Geometry check sheet. Reference: the model listing, model coordinates, mm. Face numbers are marked on the shaded views. A direction names the side the tool comes from. Give positions to 0.01 mm unless a question says otherwise; leave off trailing zeros. Write each loop counter-clockwise with the first axis right and the second up, starting at its lowest first coordinate (ties: lowest second). Pieces come first, ordered by that corner, then holes. Notation, with made-up numbers: M 5.5,86.25 L 27.5,86.25 A16 ccw 27.5,100.25 Z; hole C 73.5,26.5 d11. An arc over 180 degrees is marked long. Write each question's results on one line, items separated by ' | '.
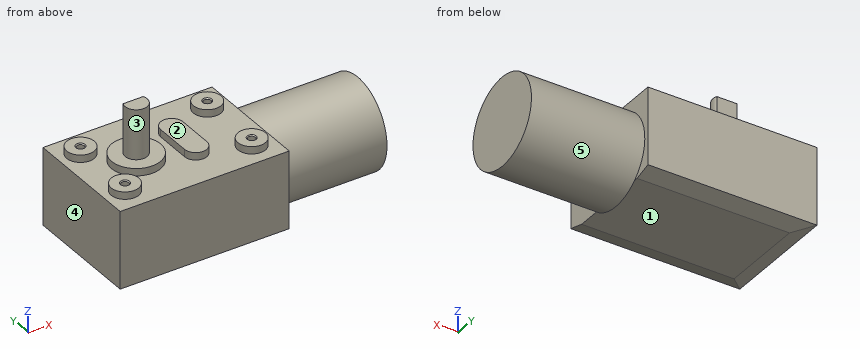
Autodesk Inventor part; units mm, degrees
ref_plane "Arbeitsebene1" through (-28.07, 15.935, 0) normal (-1, 0, 0) x (0, 0, 1)
ref_plane "YZ Plane" through (0, 0, 0) normal (1, 0, 0) x (0, 1, 0)
ref_plane "XZ Plane" through (0, 0, 0) normal (0, 1, 0) x (-1, 0, 0)
sketch "Skizze3" plane through (0, 0, 0) normal (0, 0, 1) x (1, 0, 0)
  line L0 (0, 0) -> (-45.87, 0)
  line L1 (-45.87, 0) -> (-45.87, 31.87)
  line L2 (-45.87, 31.87) -> (0, 31.87)
  line L3 (0, 31.87) -> (0, 0)
  circle A0 centre (-40.12, 25.12) radius 3.75
  line L4 (-6.8112, 15.935) -> (-34.2962, 15.935) construction
  circle A1 centre (-31.07, 15.935) radius 6.65
  circle A2 centre (-31.07, 15.935) radius 3
  circle A3 centre (-40.12, 6.75) radius 3.75
  circle A4 centre (-5.75, 25.12) radius 3.75
  circle A5 centre (-5.75, 6.75) radius 3.75
  line L5 (-18.15, 11) -> (-18.15, 20.87) construction
  line L6 (-15.15, 11) -> (-15.15, 20.87)
  line L7 (-21.15, 20.87) -> (-21.15, 11)
  arc A6 (-21.15, 11) -> (-15.15, 11) centre (-18.15, 11) ccw
  arc A7 (-15.15, 20.87) -> (-21.15, 20.87) centre (-18.15, 20.87) ccw
  point P0 (0, 15.935)
  point P1 (-18.15, 15.935)
  point P2 (-18.15, 23.87)
  point P3 (-18.15, 8)
  dimension "d5" = 6.75
  dimension "d6" = 5.75
  dimension "d7" = 7.5
  dimension "d9" = 45.87
  dimension "d10" = 31.87
  dimension "d11" = 14.8
  dimension "d12" = 13.3
  dimension "d13" = 6
  dimension "d14" = 6.75
  dimension "d15" = 6.75
  dimension "d16" = 6.75
  dimension "d17" = 5.75
  dimension "d18" = 5.75
  dimension "d19" = 5.75
  dimension "d20" = 7.5
  dimension "d21" = 7.5
  dimension "d22" = 7.5
  dimension "d23" = 15.87
  dimension "d24" = 18.15
  dimension "d25" = 6
extrude "Extrusion3" add sketch "Skizze3" against normal blind 22.25 contours L0 L1 L2 L3 | A0 | A1 | A2 | A3 | A4 | A5 | A6 L7 A7 L6
extrude "Extrusion4" add sketch "Skizze3" along normal blind 2 contours A0 | A1 | A3 | A4 | A5 | A6 L7 A7 L6
extrude "Extrusion5" add sketch "Skizze3" along normal blind 15.5 contours A2
sketch "Skizze4" plane through (0, 0, 0) normal (1, 0, 0) x (0, 0, -1)
  line L0 (0, 31.87) -> (22.25, 31.87)
  line L1 (0, 0) -> (0, 31.87)
  circle A0 centre (13.075, 18.495) radius 12.075
  dimension "d33" = 13.375
  dimension "d34" = 13.075
  dimension "d35" = 24.15
extrude "Extrusion6" add sketch "Skizze4" along normal blind 30.75
sketch "Skizze5" plane through (-5.75, 25.12, 2) normal (0, 0, 1) x (1, 0, 0)
  circle A0 centre (-34.37, 0) radius 3.75
  circle A1 centre (-34.37, -18.37) radius 3.75
  circle A2 centre (0, -18.37) radius 3.75
  circle A3 centre (0, 0) radius 3.75
  circle A4 centre (0, -18.37) radius 3.75
  point P0 (5.75, -25.12)
hole "Bohrung1" at (-5.75, 25.12, 2) at (-5.75, 6.75, 2) at (-40.12, 6.75, 2) at (-40.12, 25.12, 2) direction (0, 0, -1) diameter 2.013 depth 4.15 tip angle 118
ref_plane "Arbeitsebene1" through (-28.07, 15.935, 0) normal (-1, 0, 0) x (0, 0, 1)
sketch "Skizze6" plane through (-28.07, 15.935, 0) normal (-1, 0, 0) x (0, 0, 1)
  line L0 (15.5, -3) -> (15.5, 3)
  line L1 (2, 3) -> (15.5, 3)
  line L2 (15.5, 3) -> (3.5, 3)
  line L3 (3.5, 3) -> (3.5, 1.25)
  line L4 (3.5, 1.25) -> (15.5, 1.25)
  line L5 (15.5, 1.25) -> (15.5, 3)
  point P0 (0, -15.935)
  point P1 (3.5, 3)
  point P2 (3.5, 2.125)
  dimension "d49" = 12
  dimension "d50" = 1.75
extrude "Extrusion7" cut sketch "Skizze6" along normal blind 30.75 and the other way blind 15.375
chamfer "Fase1" distance 0.25 angle 45 4 edges at (-40.12, 7.7565, 2) (-5.75, 7.7565, 2) (-40.12, 26.1265, 2) (-5.75, 26.1265, 2)
chamfer "Fase2" distance 4.5 distance2 1.25 3 edges at (-22.935, 31.87, -22.25) (-45.87, 15.935, -22.25) (-22.935, 0, -22.25) measured on face at (-30.58, 14.1716, -22.25)
equation "\"d7\" = schraube_d"
equation "\"d9\" = gh_l"
equation "\"d10\" = gh_b"
equation "\"d12\" = s_d_u"
equation "\"d13\" = s_d"
equation "\"d20\" = d7"
equation "\"d21\" = d7"
equation "\"d22\" = d7"
equation "\"d24\" = nut_p_x_neg"
equation "\"d25\" = nut_b"
equation "\"d26\" = gh_h"
equation "\"d28\" = Absatz_h"
equation "\"d30\" = s_h"
equation "\"d35\" = M_d"
equation "\"d36\" = M_l"
equation "\"d45\" = M_l"
equation "\"s_h\" = 15.5"
equation "\"schraube_p_x\" = 6.75"
equation "\"s_p_y\" = 14.8"
equation "\"Absatz_h\" = 2"
equation "\"schraube_d\" = 7.5"
equation "\"gh_h\" = 22.25"
equation "\"M_d\" = 24.15"
equation "\"s_d\" = 6"
equation "\"M_l\" = 30.75"
equation "\"schraube_p_y\" = 5.75"
equation "\"s_d_u\" = 13.3"
equation "\"gs_h\" = 37.75"
equation "\"gh_l\" = 45.87"
equation "\"gh_b\" = 31.87"
equation "\"nut_p_x_neg\" = 18.15"
equation "\"nut_l\" = 15.87"
equation "\"nut_b\" = 6"
equation "\"m_p_z_neg\" = 13.075"
equation "\"m_p_xn\" = 13.375"
equation "\"Zet_KluppenDicke\" = 1"
equation "\"St_kurz_Höhe\" = 7.5"
equation "\"Druck_teil_Höhe\" = 7.5"
equation "\"Zet_Höhe\" = 5"
equation "\"Zet_Kluppen_Höhe\" = 7"
equation "\"Gel_Mot_St_1\" = 35"
equation "\"GM_Platte_Höhe\" = 4"
equation "\"SM_Scheibe_Durchmesser\" = 22"
equation "\"SM_Schrauben_Pos_Abstand\" = 31"
equation "\"Gel_Mot_St_Höhe\" = 5"
equation "\"Gel_Mot_St_2\" = 35"
equation "\"Bas_Haupt_Plat_Höhe\" = 4"
properties part number "BT001_trajan20_21"
Q1. Section check D-D (x = -31.07). Enter the section's corners in (y, z) (3 decimals), then the cut area to 3 significant figures.
Answer key:
outline: M 0,-21 L 4.5,-22.25 L 27.37,-22.25 L 31.87,-21 L 31.87,0 L 22.585,0 L 22.585,2 L 18.935,2 L 18.935,3.5 L 17.185,3.5 L 17.185,15.5 L 12.935,15.5 L 12.935,2 L 9.285,2 L 9.285,0 L 0,0 Z | area: 790 mm2
Q2. Section check B-B (z = -7). Enter the section's corners in (x, y).
Answer key:
outline: M -45.87,0 L 0,0 L 0,8.06 L 30.75,8.06 L 30.75,28.93 L 0,28.93 L 0,31.87 L -45.87,31.87 Z
Q3. Section check C-C (y = 14.5). Enter the section's corners in (x, z).
Answer key:
outline: M -45.87,-21 L -41.37,-22.25 L 0,-22.25 L 0,-24.47 L 30.75,-24.47 L 30.75,-1.68 L 0,-1.68 L 0,0 L -15.15,0 L -15.15,2 L -21.15,2 L -21.15,0 L -24.58,0 L -24.58,2 L -28.44,2 L -28.44,15.5 L -33.7,15.5 L -33.7,2 L -37.56,2 L -37.56,0 L -45.87,0 Z
Q4. Access from +Z, -Z, +X, -X, +Y, -Y to the whole of each face (thin tool, end or side, straight path). Record for the marked faces 1, 2, 3, 4 and 5.
Answer key:
face 1: -Z, -X, +Y, -Y | face 2: +Z, +X, +Y, -Y | face 3: +Z | face 4: +Z, -Z, -X, +Y, -Y | face 5: +X
Q5. Section check A-A (x = -18.15). Enter the section's corners in (y, z).
Answer key:
outline: M 0,-21 L 4.5,-22.25 L 27.37,-22.25 L 31.87,-21 L 31.87,0 L 23.87,0 L 23.87,2 L 8,2 L 8,0 L 0,0 Z
Q6. Depth check by flat-ended pin: P1, Ø10, axis at x = 9, y = 15, coming from the +Z side; P2, Ø4, axis at x = -42, y = 26.5, coming from the +Z side; P3, Ø2.5, axis at x = -40.12, y = 25.12, coming from the -Z side; P4, Ø2, axis at x = -19, z = -11.5, coming from the -Y side. Enter the tip coordinate at first touch or a pass-through.
Answer key:
P1: stops at z = -1 | P2: stops at z = 2 | P3: stops at z = -22.25 | P4: stops at y = 0
Q7. Material ranges on probe 1 along X at (y, z) = (6.75, -0.5); probe 2 along Y at (x, z) = (-5.75, -1.1); probe 3 along X at (y, z) = (6.5, -17), recorded low to high. Write a range as [from, to].
Answer key:
probe 1: x = [-45.87, -41.13], [-39.11, -6.76], [-4.74, 0] | probe 2: y = [0, 5.74], [7.76, 24.11], [26.13, 31.87] | probe 3: x = [-45.87, 0]
